The figure shows three views and two pictorial views of one solid part (mm, origin at its lowest corner). Answer the questions. Coordinates: 2 decimals unless noted, no trailing zeros. Order: outer loops, then holes, each group sorted by start corner. A loop starts at its lowest first (then second) coordinate and runs counter-clockwise, first axis right, second up. Notation, with made-up numbers: (57, 19) -> (109, 19) arc R4 ccw to (109, 26) -> close; hole circle Ø11 at (18.25, 54.25). An arc over 180 degrees is marked (long way). Write item = value, one per line. Start each with the question number.
Q1. Straight lines are drawn through the part: L1, parallel to Y at x = 100, z = 4; L2, parallel to X at y = 7.5, z = 22; L3, parallel to Y at x = 102, z = 17. For each, find the intervals that lie inside material, in ascending order. Write a range as from..to.
Q2. The part is cut by section A-A, the plane z = 9. Determine the outline of the cut face in (x, y), plus the area to 3 significant figures.
Q3. Flat-ended cylindrical pins translate along their axes: pin 1 (2.5 mm diameter, centred on x = 100.5, y = 25, fed in from -Z); pin 2 (10 mm diameter, centred on x = 25, z = 25, fed in from -Y). Find the tip coordinate at first contact, or state that the pin passes through.
Q4. The part is cut by section C-C, the plane x = 105. Determine the outline of the cut face in (y, z).
Q5. For a pull along X with two mould halves and no side action, classify the marked faces 1, 2 and 3 as +X half, -X half, draft (parallel to the pull), parting line (faces both ways), or undercut.
Q6. The part is cut by section B-B, the plane y = 15. Determine the outline of the cut face in (x, z).
Q7. The part is cut by section D-D, the plane z = 25. Determine the outline of the cut face in (x, y), plus the area to 3 significant figures.
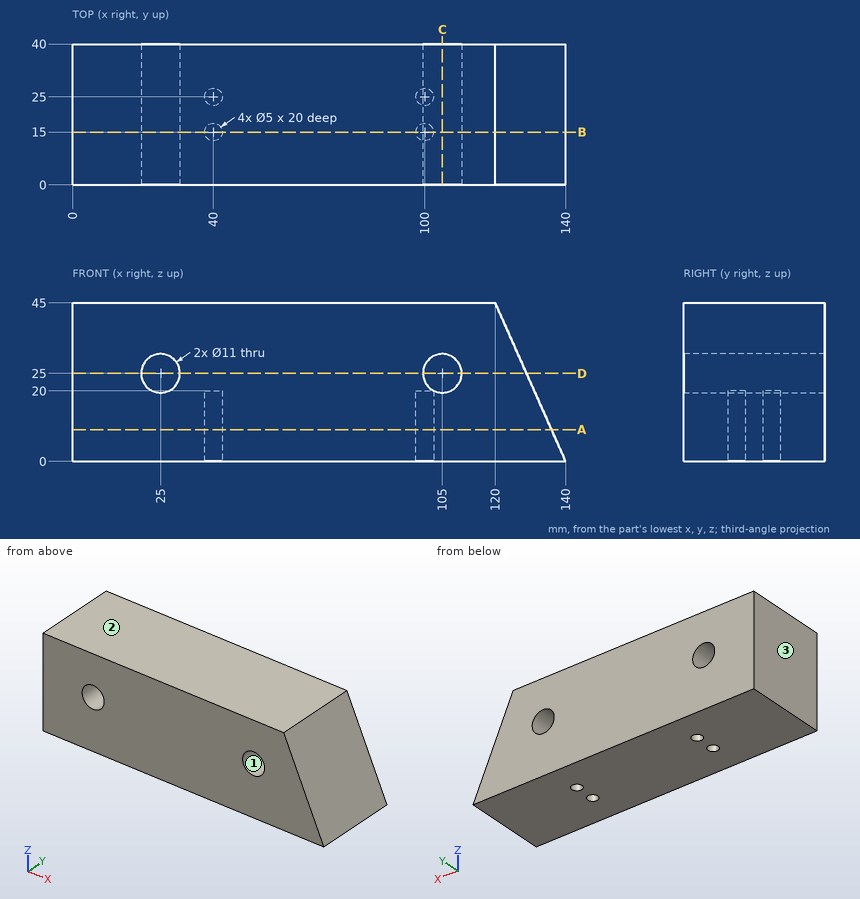
Model answer:
q1.L1 = 0..12.5, 17.5..22.5, 27.5..40
q1.L2 = 0..20.39, 29.61..100.39, 109.61..130.22
q1.L3 = 0..13.5, 16.5..23.5, 26.5..40
q2.outline = (0, 0) -> (136, 0) -> (136, 40) -> (0, 40) -> close; hole circle Ø5 at (40, 15); hole circle Ø5 at (40, 25); hole circle Ø5 at (100, 15); hole circle Ø5 at (100, 25)
q2.area = 5,360 mm2
q3.pin_1 = 20
q3.pin_2 = through
q4.outline = (0, 0) -> (40, 0) -> (40, 19.5) -> (0, 19.5) -> close; (0, 30.5) -> (40, 30.5) -> (40, 45) -> (0, 45) -> close
q5.face_1 = undercut
q5.face_2 = draft
q5.face_3 = -X half
q6.outline = (0, 0) -> (37.5, 0) -> (37.5, 20) -> (42.5, 20) -> (42.5, 0) -> (97.5, 0) -> (97.5, 20) -> (102.5, 20) -> (102.5, 0) -> (140, 0) -> (120, 45) -> (0, 45) -> close; hole circle Ø11 at (25, 25); hole circle Ø11 at (105, 25)
q7.outline = (0, 0) -> (19.5, 0) -> (19.5, 40) -> (0, 40) -> close; (30.5, 0) -> (99.5, 0) -> (99.5, 40) -> (30.5, 40) -> close; (110.5, 0) -> (128.89, 0) -> (128.89, 40) -> (110.5, 40) -> close
q7.area = 4,280 mm2
